Check sheet for the modelled part. Datum: model origin and axes. Units: mm. A direction names the side the tool comes from. Coordinates: 2 decimals unless noted, no trailing zeros. Write each loop counter-clockwise with the first axis right and the second up, starting at its lowest first coordinate (ties: lowest second). Pieces come first, ordered by that corner, then holes. Notation, with made-up numbers: M -13.75,53.5 L 36.25,53.5 A21 cw 36.25,67.5 Z; hole C -24.5,38.25 d7. An arc over 180 degrees is marked long. Answer as CSV lines item,"result". Start each with the question number.
1) Material ranges on L1, parallel to X at y = 0.25, z = 3; L2, parallel to Z at x = 9, y = 13.5; L3, parallel to Y at x = 2, z = 1.8, recorded low to high. Write a range as [from, to].
2) Section check D-D (y = -9). Record the cut outline in (x, z).
3) Section check C-C (x = 3.5). Record the cut outline in (y, z), and give its area (3 significant figures).
4) Access from +Z, -Z, +X, -X, +Y, -Y to the whole of each face (thin tool, end or side, straight path). Record for faces 1 (the flat face through (-4, -12, 1)), 2 (the cylindrical face through (9.745, -35.361, 2.535)).
5) Go/stop test with flat-tipped pins: pin 1 Ø2 at (x, z) = (-7.5, 2.5) entering from +Y; pin 2 Ø7 at (x, y) = (-3.5, 3) entering from -Z; pin 3 Ø3.5 at (x, y) = (4.5, -24.5) entering from -Z. Record where each tip stops, or that it passes through.
6) Section check B-B (z = 4.3). Record the cut outline in (x, y), and give its area (3 significant figures).
7) Draft check along Y on faces 3 (the cylindrical face through (4.142, 27.977, 3.521)), 4 (the flat face through (0, -24, 0)), 5 (the cylindrical face through (-9.861, -35.245, 2.535)). Enter one of: +Y half, -Y half, draft (parallel to the pull), parting line (faces both ways), or undercut.
8) Section check A-A (y = 0.25). Record the cut outline in (x, z), and give its area (3 significant figures).
from build123d import *

# Parameters (mm, degrees)
F0_W     = 24
F0_H     = 75
F1_DEPTH = 5
F2_R     = 2.75
F2_R_2   = 2
F3_DEPTH = 5
F4_R     = 7.5
F5_R     = 2.75
F6_DEPTH = 2


with BuildPart() as f1:
    # F0 (on Top) → F1 (new body)
    with BuildSketch(Plane.XY):
        Rectangle(F0_W, F0_H)
    extrude(amount=F1_DEPTH)

    # F2 (on face) → F3 (cut)
    with BuildSketch(Plane.XY.offset(5)):
        with Locations((4.5, 25.25)):
            Circle(F2_R)
        with Locations((4.5, 0.25)):
            Circle(F2_R)
        with Locations((4.5, -24.5)):
            Circle(F2_R_2)
    extrude(amount=-F3_DEPTH, mode=Mode.SUBTRACT)

    # F4
    f4_edges = [f1.edges().sort_by_distance(p)[0] for p in [
        (12, 37.5, 2.5),
        (-12, 37.5, 2.5),
        (12, -37.5, 2.5),
        (-12, -37.5, 2.5),
    ]]
    fillet(f4_edges, radius=F4_R)

    # F5 (on face) → F6 (cut)
    with BuildSketch(Plane(origin=(0, 0, 0), x_dir=(1, 0, 0), z_dir=(0, 0, -1))):
        with BuildLine():
            Line((4.5, 12), (-12, 12))
            Line((-12, 12), (-12, -30))
            ThreePointArc((-12, -30), (-9.803301, -35.303301), (-4.5, -37.5))
            Line((-4.5, -37.5), (4.5, -37.5))
            ThreePointArc((4.5, -37.5), (9.803301, -35.303301), (12, -30))
            Line((12, -30), (12, 4.5))
            ThreePointArc((12, 4.5), (9.803301, 9.803301), (4.5, 12))
        make_face()
        with Locations((4.5, -25.25)):
            Circle(F5_R, mode=Mode.SUBTRACT)
        with Locations((4.5, -0.25)):
            Circle(F5_R, mode=Mode.SUBTRACT)
    extrude(amount=-F6_DEPTH, mode=Mode.SUBTRACT)


solid = f1.part
Results found:
1,L1,"x = [-12, 1.75], [7.25, 12]"
1,L2,"z = [2, 5]"
1,L3,"y = [-37.5, -12]"
2,outline,"M -12,2 L 10.5,2 L 10.5,0 L 12,0 L 12,5 L -12,5 Z"
3,outline,"M -37.5,0 L -26.23,0 L -26.23,5 L -37.5,5 Z; M -22.77,0 L -12,0 L -12,2 L -2.31,2 L -2.31,5 L -22.77,5 Z; M 2.81,2 L 22.69,2 L 22.69,5 L 2.81,5 Z; M 27.81,2 L 37.5,2 L 37.5,5 L 27.81,5 Z"
3,area,"228 mm2"
4,face 1,"-Z, -X, +Y"
4,face 2,"+Z, -Z, +X, -Y"
5,pin 1,"stops at y = 37.23"
5,pin 2,"stops at z = 2"
5,pin 3,"passes through"
6,outline,"M -12,-30 A7.5 ccw -4.5,-37.5 L 4.5,-37.5 A7.5 ccw 12,-30 L 12,30 A7.5 ccw 4.5,37.5 L -4.5,37.5 A7.5 ccw -12,30 Z; hole C 4.5,0.25 d5.5; hole C 4.5,25.25 d5.5; hole C 4.5,-24.5 d4"
6,area,"1,690 mm2"
7,face 3,"undercut"
7,face 4,"draft"
7,face 5,"-Y half"
8,outline,"M -12,2 L 1.75,2 L 1.75,5 L -12,5 Z; M 7.25,2 L 12,2 L 12,5 L 7.25,5 Z"
8,area,"55.5 mm2"
